Here's how the part is built. I have some questions about the finished solid (model axes, mm). A direction names the side the tool comes from. Give positions to 0.01 mm unless a question says otherwise; leave off trailing zeros. Loops run counter-clockwise (first coordinate to the right, second up) from the corner with the lowest first, then second, coordinate; pieces in that order, holes last.
Q1. I'm going to push flat-ended pins straight in: P1, Ø1.8, axis at x = 0, y = 22.5, coming from the +Z side; P2, Ø1.3, axis at x = -1, y = 0, coming from the +Z side. Where does each tip first touch, or does it pass through?
Q2. Suppose I cut it at A-A (x = -5.75). List the corners of the cut face in (y, z) for me, and give its area (3 significant figures).
Q3. Suppose I cut it at C-C (z = 6.5). List the corners of the cut face in (x, y) for me, and give its area (3 significant figures).
Q4. Suppose I cut it at B-B (y = -22.5). List the corners of the cut face in (x, z) for me.
Q5. Thinking about a two-plate mould opening in X: for faces 4 (the face through (0, -14, 10)), 5 (the face through (1.45, -13, 5)), 6 (the face through (0, -21, 5)), 7 (the face through (9, 0, 4)), which applies, pulls with the +X half, pulls with the -X half, needs draft (parallel to the pull), parting line crosses it, or undercut?
Q6. Suppose I cut it at D-D (x = 0). List the corners of the cut face in (y, z) for me, and give its area (3 significant figures).
Q7. I need wall thicknesses on probe 1 along Y at (x, z) = (0, 8.25); probe 2 along Y at (x, z) = (-2, 8.5); probe 3 along Y at (x, z) = (-0.75, 2.5). Which ranges of each line are inside material? Lowest first, please.
Q8. For faces 1 (the face through (0, -1, 7)), 2 (the face through (0, 24, 5)), 3 (the face through (-4, -11.5, 5)), which set-ups out of +Z, -Z, +X, -X, +Y, -Y let a thin tool reach every point of the face, with its end or its side?
Autodesk Inventor part; units mm, degrees
ref_plane "YZ Plane" through (0, 0, 0) normal (1, 0, 0) x (0, 1, 0)
ref_plane "XZ Plane" through (0, 0, 0) normal (0, 1, 0) x (-1, 0, 0)
ref_plane "XY Plane" through (0, 0, 0) normal (0, 0, 1) x (1, 0, 0)
sketch "スケッチ1" plane through (0, 0, 0) normal (0, 0, 1) x (1, 0, 0)
  line L0 (-9, -27.5) -> (9, -27.5)
  line L1 (9, -27.5) -> (9, 27.5)
  line L2 (9, 27.5) -> (-9, 27.5)
  line L3 (-9, 27.5) -> (-9, -27.5)
  line L4 (-9, -27.5) -> (9, 27.5) construction
  line L5 (9, -27.5) -> (-9, 27.5) construction
  point P0 (0, 0)
  dimension "d0" = 18
  dimension "d1" = 55
extrude "押し出し1" add sketch "スケッチ1" along normal blind 10
sketch "スケッチ2" plane through (0, 0, 10) normal (0, 0, 1) x (1, 0, 0)
  line L0 (-9, 27.5) -> (-9, -27.5)
  line L1 (9, -27.5) -> (9, 27.5)
  line L2 (-9, -1) -> (9, -1)
  line L3 (9, -1) -> (9, 1.6)
  line L4 (9, 1.6) -> (-9, 1.6)
  line L5 (-9, 1.6) -> (-9, -1)
  line L6 (-9, -27.5) -> (9, -27.5)
  point P0 (0, 0)
  point P1 (9, -1)
  dimension "d4" = 2.6
  dimension "d5" = 26.5
extrude "押し出し2" cut sketch "スケッチ2" against normal blind 5.5 contours L4 L1 L2 L0
sketch "スケッチ3" plane through (0, 0, 10) normal (0, 0, 1) x (1, 0, 0)
  line L0 (-9, -1) -> (-9, -27.5)
  line L1 (-9, -13.5) -> (1.45, -13.5)
  line L2 (1.45, -13.5) -> (1.45, -11.5)
  line L3 (1.45, -11.5) -> (-9, -11.5)
  line L4 (-9, -11.5) -> (-9, -13.5)
  line L5 (-9, -27.5) -> (9, -27.5)
  point P0 (0, 0)
  dimension "d8" = 2
  dimension "d9" = 14
  dimension "d10" = 10.45
extrude "押し出し3" cut sketch "スケッチ3" against normal through all
sketch "スケッチ4" plane through (0, 0, 10) normal (0, 0, 1) x (1, 0, 0)
  circle A0 centre (0, 22.5) radius 1.5
  circle A1 centre (0, -22.5) radius 1.5
  line L0 (9, 27.5) -> (-9, 27.5)
  line L1 (-9, -27.5) -> (9, -27.5)
  point P0 (0, 0)
  dimension "d13" = 3
  dimension "d14" = 3
  dimension "d15" = 5
  dimension "d16" = 5
extrude "押し出し4" cut sketch "スケッチ4" against normal through all
properties part number "ジョイントモーターハメ"
Solutions:
1. P1: passes through
1. P2: stops at z = 4.5
2. outline: (-27.5, 0) - (-13.5, 0) - (-13.5, 10) - (-27.5, 10) - close; (-11.5, 0) - (27.5, 0) - (27.5, 10) - (1.6, 10) - (1.6, 4.5) - (-1, 4.5) - (-1, 10) - (-11.5, 10) - close
2. area: 516 mm2
3. outline: (-9, -27.5) - (9, -27.5) - (9, -1) - (-9, -1) - (-9, -11.5) - (1.45, -11.5) - (1.45, -13.5) - (-9, -13.5) - close; (-9, 1.6) - (9, 1.6) - (9, 27.5) - (-9, 27.5) - close; hole circle Ø3 at (0, -22.5); hole circle Ø3 at (0, 22.5)
3. area: 908 mm2
4. outline: (-9, 0) - (-1.5, 0) - (-1.5, 10) - (-9, 10) - close; (1.5, 0) - (9, 0) - (9, 10) - (1.5, 10) - close
5. face 4: needs draft
5. face 5: pulls with the -X half
5. face 6: undercut
5. face 7: pulls with the +X half
6. outline: (-27.5, 0) - (-24, 0) - (-24, 10) - (-27.5, 10) - close; (-21, 0) - (-13.5, 0) - (-13.5, 10) - (-21, 10) - close; (-11.5, 0) - (21, 0) - (21, 10) - (1.6, 10) - (1.6, 4.5) - (-1, 4.5) - (-1, 10) - (-11.5, 10) - close; (24, 0) - (27.5, 0) - (27.5, 10) - (24, 10) - close
6. area: 456 mm2
7. probe 1: y = -27.5 to -24, -21 to -13.5, -11.5 to -1, 1.6 to 21, 24 to 27.5
7. probe 2: y = -27.5 to -13.5, -11.5 to -1, 1.6 to 27.5
7. probe 3: y = -27.5 to -23.8, -21.2 to -13.5, -11.5 to 21.2, 23.8 to 27.5
8. face 1: +Z, +X, -X
8. face 2: +Z, -Z
8. face 3: +Z, -Z, -X
